For this review, take the finished solid that the model builds, in its own axes (mm). Face numbers are marked on the shaded views. Coordinates: 2 decimals unless noted, no trailing zeros. Write each loop counter-clockwise with the first axis right and the second up, starting at its lowest first coordinate (ties: lowest second). Pieces come first, ordered by that corner, then holes. Notation, with made-up numbers: M 69.25,29 L 104.25,29 A30 ccw 104.25,54 Z; hole C -29.5,87 d8. An arc over 180 degrees is marked long. Return JSON: item names as keys, results as strings.
```python
from build123d import *

# Parameters (mm, degrees)
SKETCH1_W           = 50
SKETCH1_H           = 22
BOSS_EXTRUDE1_DEPTH = 60
CUT_EXTRUDE2_REACH  = 125.069
CUT_EXTRUDE3_REACH  = 125.069
SKETCH6_R           = 6.26
FILLET1_R           = 5
SKETCH2_R           = 2.5
BOSS_EXTRUDE2_DEPTH = 10
LPATTERN1_COUNT     = 6
LPATTERN1_PITCH     = 20
SKETCH3_R           = 2.5
BOSS_EXTRUDE3_DEPTH = 10
LPATTERN2_COUNT     = 6
LPATTERN2_PITCH     = 20
SKETCH4_R           = 7
CUT_EXTRUDE1_DEPTH  = 30


with BuildPart() as part:
    # Sketch1 → Boss-Extrude1 (new, symmetric)
    with BuildSketch(Plane(origin=(0, 0, 0), x_dir=(0, 0, -1), z_dir=(1, 0, 0))):
        Rectangle(SKETCH1_W, SKETCH1_H)
    extrude(amount=BOSS_EXTRUDE1_DEPTH, both=True)

    # Sketch5 → Cut-Extrude2 (cut, up to next)
    with BuildSketch(Plane(origin=(60, 0, 0), x_dir=(0, 0, -1), z_dir=(1, 0, 0)), mode=Mode.PRIVATE) as cut_extrude2_sk1:
        with BuildLine():
            Line((-26.243342576, 11), (-23.75, 11))
            Line((-23.75, 11), (-23.75, 6.005))
            ThreePointArc((-23.75, 6.005), (-35.592030441, 3.213639122), (-26.243342576, 11))
        make_face()
    cut_extrude2_tool1 = extrude(cut_extrude2_sk1.sketch, amount=-CUT_EXTRUDE2_REACH, mode=Mode.PRIVATE) & part.part
    add(cut_extrude2_tool1.solids().sort_by_distance((60, 6.117758, 29.835764))[0], mode=Mode.SUBTRACT)

    # Sketch6 → Cut-Extrude3 (cut, up to next)
    with BuildSketch(Plane.ZY.offset(60), mode=Mode.PRIVATE) as cut_extrude3_sk1:
        with Locations((30, -6.005)):
            Circle(SKETCH6_R)
    cut_extrude3_tool1 = extrude(cut_extrude3_sk1.sketch, amount=-CUT_EXTRUDE3_REACH, mode=Mode.PRIVATE) & part.part
    add(cut_extrude3_tool1.solids().sort_by_distance((-60, -6.005, 30))[0], mode=Mode.SUBTRACT)

    # Fillet1
    fillet1_edges = [part.edges().sort_by_distance(p)[0] for p in [
        (0, 11, 23.75),
    ]]
    fillet(fillet1_edges, radius=FILLET1_R)

    # Sketch2 → Boss-Extrude2 (add)
    with BuildSketch(Plane(origin=(60, 0, 0), x_dir=(0, 0, -1), z_dir=(1, 0, 0))):
        with BuildLine():
            Line((-30, 1.202041029), (-18.75, 1.202041029))
            Line((-18.75, 1.202041029), (-18.75, 11))
            Line((-18.75, 11), (-30, 11))
            ThreePointArc((-30, 11), (-34, 6.101020514), (-30, 1.202041029))
        make_face()
        with Locations((-29, 6.101020514)):
            Circle(SKETCH2_R, mode=Mode.SUBTRACT)
    boss_extrude2 = extrude(amount=-BOSS_EXTRUDE2_DEPTH)

    # LPattern1: Boss-Extrude2 ×6
    with Locations(*[(-i * LPATTERN1_PITCH, 0, 0) for i in range(1, LPATTERN1_COUNT)]):
        add(boss_extrude2)

    # Sketch3 → Boss-Extrude3 (add)
    with BuildSketch(Plane.ZY.offset(60)):
        with BuildLine():
            Line((23.75, -1.202041029), (30, -1.202041029))
            ThreePointArc((30, -1.202041029), (34, -6.101020514), (30, -11))
            Line((30, -11), (23.75, -11))
            Line((23.75, -11), (23.75, -1.202041029))
        make_face()
        with Locations((29, -6.101020514)):
            Circle(SKETCH3_R, mode=Mode.SUBTRACT)
    boss_extrude3 = extrude(amount=-BOSS_EXTRUDE3_DEPTH)

    # LPattern2: Boss-Extrude3 ×6
    with Locations(*[(i * LPATTERN2_PITCH, 0, 0) for i in range(1, LPATTERN2_COUNT)]):
        add(boss_extrude3)

    # Sketch4 → Cut-Extrude1 (cut)
    with BuildSketch(Plane(origin=(0, 0, -25), x_dir=(-1, 0, 0), z_dir=(0, 0, -1))):
        with Locations(Location((0, 0, 0), (0, 0, 90))):
            Circle(SKETCH4_R)
    extrude(amount=-CUT_EXTRUDE1_DEPTH, mode=Mode.SUBTRACT)


solid = part.part
```
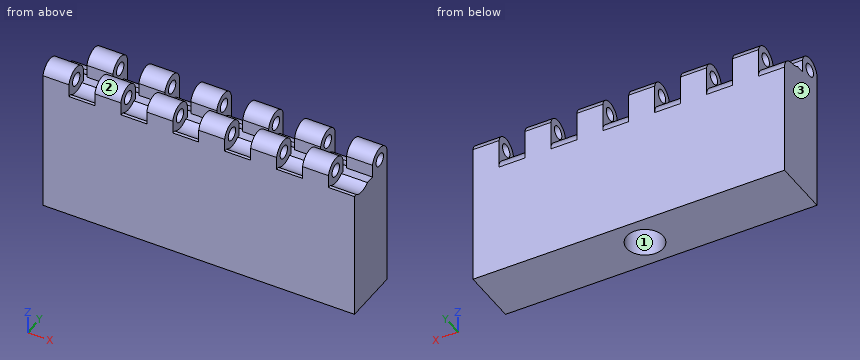
1. We need section B-B (z = -8). State the section outline as (x, y) points, plus the area to 3 significant figures.
Checks:
{"outline": "M -60,-11 L 60,-11 L 60,11 L -60,11 Z; hole C 0,0 d14", "area": "2,490 mm2"}
2. Wall thickness on L1, parallel to X at y = -5.25, z = 25; L2, parallel to Y at x = 37, z = 29; L3, parallel to Y at x = 26, z = 29: over which ranges is each line inside the solid? List them lowest first. Write a range as from..to.
Checks:
{"L1": "-60..-50, -40..-30, -20..-10, 0..10, 20..30, 40..50", "L2": "1.2..3.6, 8.6..11", "L3": "-11..-8.6, -3.6..-1.2"}
3. Clearance check with flat-ended pins moving along their axes: pin 1 Ø2.5 at (x, z) = (25.5, 27.5) entering from +Y; pin 2 Ø3 at (y, z) = (8.5, 27.5) entering from -X; pin 3 Ø6.5 at (y, z) = (-6.1, 29) entering from +X. State where each tip first meets the part, or that it passes through.
Checks:
{"pin 1": "y = -1.2", "pin 2": "x = -50", "pin 3": "x = 50"}
4. We need section C-C (x = 34). State the section outline as (y, z) points (3 decimals).
Checks:
{"outline": "M -11,-25 L 11,-25 L 11,30 A5 ccw 1.202,30 L 1.202,25 L -2.238,25 A6.26 cw -9.772,25 L -11,25 Z; hole C 6.101,29 d5"}
5. Draft analysis for pull direction X (two halves, no side actions). For the marked faces 1, 2 and 3, state which applies: +X half, -X half, draft (parallel to the pull), parting line (faces both ways), or undercut.
Checks:
{"face 1": "undercut", "face 2": "draft", "face 3": "-X half"}
6. We need section A-A (y = 0). State the section outline as (x, z) points, plus the area to 3 significant figures.
Checks:
{"outline": "M -60,-25 L -7,-25 L -7,5 L 7,5 L 7,-25 L 60,-25 L 60,25 L -60,25 Z", "area": "5,580 mm2"}
